Work out the finished part from the listing and answer in its coordinate system (mm). A direction names the side the tool comes from. Round coordinates to 2 decimals unless told otherwise and drop trailing zeros. Loops run counter-clockwise (first coordinate to the right, second up) from the corner with the lowest first, then second, coordinate; pieces in that order, holes last.
from build123d import *

# Parameters (mm, degrees)
SKETCH1_W               = 24
SKETCH1_H               = 30
BOSS_EXTRUDE1_DEPTH     = 60
CUT_EXTRUDE1_DEPTH      = 25
CUT_EXTRUDE1_DEPTH_BACK = 1
BOSS_EXTRUDE2_DEPTH     = 52
CUT_EXTRUDE3_DEPTH      = 31
CUT_EXTRUDE3_DEPTH_BACK = 20


with BuildPart() as part:
    # Sketch1 → Boss-Extrude1 (new body)
    with BuildSketch(Plane(origin=(0, 0, 0), x_dir=(1, 0, 0), z_dir=(0, 1, 0))):
        with Locations((12, 15)):
            Rectangle(SKETCH1_W, SKETCH1_H)
    extrude(amount=BOSS_EXTRUDE1_DEPTH)

    # Sketch2 → Cut-Extrude1 (cut, two sides)
    with BuildSketch(Plane(origin=(0, 0, 0), x_dir=(0, 0, -1), z_dir=(1, 0, 0))) as cut_extrude1_sk:
        with BuildLine():
            Line((0, 60), (0, 22))
            ThreePointArc((0, 22), (2.928932188, 29.071067812), (10, 32))
            Line((10, 32), (20, 32))
            ThreePointArc((20, 32), (27.071067812, 34.928932188), (30, 42))
            Line((30, 42), (30, 60))
            Line((30, 60), (0, 60))
        make_face()
    extrude(amount=CUT_EXTRUDE1_DEPTH, mode=Mode.SUBTRACT)
    extrude(cut_extrude1_sk.sketch, amount=-CUT_EXTRUDE1_DEPTH_BACK, mode=Mode.SUBTRACT)

    # Sketch1<5> → Boss-Extrude2 (add)
    with BuildSketch(Plane(origin=(0, 0, 0), x_dir=(1, 0, 0), z_dir=(0, 1, 0))):
        Polygon((0, 50), (0, 30), (24, 30), (40, 30), (40, 50), align=None)
    extrude(amount=BOSS_EXTRUDE2_DEPTH)

    # Sketch5 → Cut-Extrude3 (cut, two sides)
    with BuildSketch(Plane.XY.offset(-30)) as cut_extrude3_sk:
        with BuildLine():
            Line((-101.427106217, 52), (20, 52))
            ThreePointArc((20, 52), (34.142135624, 46.142135624), (40, 32))
            Line((40, 32), (40, -89.427106217))
            Line((40, -89.427106217), (211.723860452, 82.296754235))
            Line((211.723860452, 82.296754235), (70.296754235, 223.723860452))
            Line((70.296754235, 223.723860452), (-101.427106217, 52))
        make_face()
    extrude(amount=CUT_EXTRUDE3_DEPTH, mode=Mode.SUBTRACT)
    extrude(cut_extrude3_sk.sketch, amount=-CUT_EXTRUDE3_DEPTH_BACK, mode=Mode.SUBTRACT)


solid = part.part
Item 1: Straight lines are drawn through the part: line 1 (X direction, y = 28, z = -28.5); line 2 (Z direction, x = 8.5, y = 48); line 3 (Y direction, x = 20, z = -16.5). For each, find the intervals that lie inside material, in ascending order.
Item 2: For faces 1 (the face through (12, 32, -15)), 2 (the face through (24, 16, -15)), 3 (the face through (20, 26, -50)), 4 (the face through (24.2, 31.4, -30)), determine the directions among +Z, -Z, +X, -X, +Y, -Y from which every point of the face is accessible in a straight line to the end or side of a thin tool.
Item 3: Section D-D, the plane y = 38 is taken. Give the vertices of the cut face in (x, z).
Item 4: Section C-C, the plane z = -40 is taken. Give the vertices of the cut face in (x, y).
Item 5: Section A-A, the plane x = 8 is taken. Give the vertices of the cut face in (y, z).
Item 6: Section B-B, the plane y = 6.5 is taken. Give the vertices of the cut face in (x, z).
Item 7: Each of these flat-tipped pins is pushed along its axis until it touches: P1, Ø6, axis at x = 26.5, z = -32.5, coming from the +Y side; P2, Ø1, axis at x = 28.5, y = 23.5, coming from the +Z side; P3, Ø3, axis at x = 6.5, z = -16, coming from the +Y side. Where does it stop, or does it pass through?
Answer below:
1. line 1: x = 0 to 24
1. line 2: z = -50 to -30
1. line 3: y = 0 to 32
2. face 1: +Z, +X, -X, +Y
2. face 2: +Z, +X, +Y, -Y
2. face 3: -Z, +X, -X, +Y, -Y
2. face 4: +Z, +X, +Y
3. outline: (0, -50) - (39.08, -50) - (39.08, -30) - (24, -30) - (24, -29.17) - (0, -29.17) - close
4. outline: (0, 0) - (40, 0) - (40, 32) arc R20 ccw to (20, 52) - (0, 52) - close
5. outline: (0, -50) - (52, -50) - (52, -30) - (42, -30) arc R10 cw to (32, -20) - (32, -10) arc R10 ccw to (22, 0) - (0, 0) - close
6. outline: (0, -50) - (40, -50) - (40, -30) - (24, -30) - (24, 0) - (0, 0) - close
7. P1: stops at y = 51.69
7. P2: stops at z = -30
7. P3: stops at y = 32
